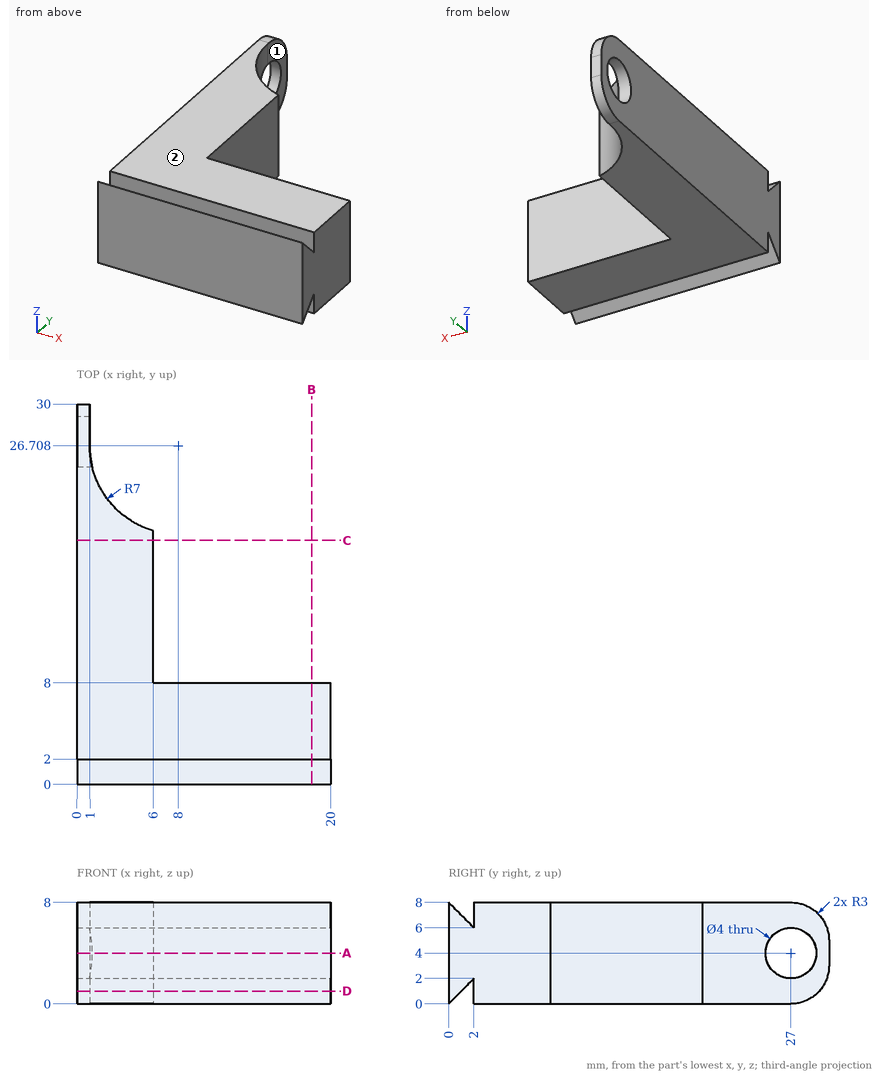
Study the drawing (mm; zero at the part's minimum x, y, z) and answer. A direction names the side the tool comes from. Coordinates: 2 decimals unless noted, no trailing zeros. Write each loop counter-clockwise with the first axis right and the second up, starting at its lowest first coordinate (ties: lowest second). Pieces come first, ordered by that corner, then holes.
Q1. Which of the six approach directions +Z, -Z, +X, -X, +Y, -Y give full straight-line access (tool end or side, diameter ignored) to the marked faces 1 and 2?
Returned:
face 1: +Z, -Z, +X, +Y
face 2: +Z, +X, -X, +Y, -Y
Q2. Section A-A, the plane z = 4 is taken. Write down the section's boundary in (x, y), then the cut area to 3 significant figures.
Returned:
outline: (0, 0) - (20, 0) - (20, 8) - (6, 8) - (6, 20) arc R7 cw to (1.21, 25) - (0, 25) - close; (0, 29) - (1, 29) - (1, 30) - (0, 30) - close
area: 247 mm2
Q3. Find the intervals of material crossed by line 1 along Y through (x, z) = (9, 1); line 2 along Y through (x, z) = (0.6, 4); line 3 along Z through (x, y) = (0.6, 27), in increasing order.
Returned:
line 1: y = 0 to 1, 2 to 8
line 2: y = 0 to 25, 29 to 30
line 3: z = 0 to 2, 6 to 8
Q4. Section B-B, the plane x = 18.5 is taken. Write down the section's boundary in (y, z).
Returned:
outline: (0, 0) - (2, 2) - (2, 0) - (8, 0) - (8, 8) - (2, 8) - (2, 6) - (0, 8) - close
Q5. Given P1, Ø2.5, axis at y = 28, z = 4, coming from the +X side, flat-ended and moving along its own axis, determine where the tip first touches the part or whether it passes through.
Returned:
P1: stops at x = 1
Q6. Section C-C, the plane y = 19.25 is taken. Write down the section's boundary in (x, z), then the cut area to 3 significant figures.
Returned:
outline: (0, 0) - (6, 0) - (6, 8) - (0, 8) - close
area: 48.0 mm2
Q7. Section D-D, the plane z = 1 is taken. Write down the section's boundary in (x, y).
Returned:
outline: (0, 0) - (20, 0) - (20, 1) - (0, 1) - close; (0, 2) - (20, 2) - (20, 8) - (6, 8) - (6, 20) arc R7 cw to (1, 26.71) - (1, 29.24) - (0, 29.24) - close
